```python
from build123d import *

# Parameters (mm, degrees)
ESQUISSE2_W              = 290
ESQUISSE2_H              = 184.53
BOSS_EXTRU_1_DEPTH       = 10
ESQUISSE9_R              = 2
ENL_V_MAT_EXTRU_7_DEPTH  = 10
ESQUISSE12_R             = 2
ENL_V_MAT_EXTRU_10_DEPTH = 10
ENL_V_MAT_EXTRU_12_DEPTH = 10
ENL_V_MAT_EXTRU_13_DEPTH = 10
CONG_1_R                 = 30
CONG_2_R                 = 30
ESQUISSE16_R             = 6
ENL_V_MAT_EXTRU_14_DEPTH = 5


with BuildPart() as part:
    # Esquisse2 → Boss.-Extru.1 (new body)
    with BuildSketch(Plane(origin=(0, 0, 0), x_dir=(1, 0, 0), z_dir=(0, 1, 0))):
        with Locations((145, 92.265)):
            Rectangle(ESQUISSE2_W, ESQUISSE2_H)
    extrude(amount=BOSS_EXTRU_1_DEPTH)

    # Esquisse9 → Enlèv. mat.-Extru.7 (cut)
    with BuildSketch(Plane(origin=(0, 10, 0), x_dir=(1, 0, 0), z_dir=(0, 1, 0))):
        with Locations((45, 50)):
            Circle(ESQUISSE9_R)
        with Locations((245, 50)):
            Circle(ESQUISSE9_R)
    extrude(amount=-ENL_V_MAT_EXTRU_7_DEPTH, mode=Mode.SUBTRACT)

    # Esquisse12 → Enlèv. mat.-Extru.10 (cut)
    with BuildSketch(Plane.XZ):
        with Locations((10, -165)):
            Circle(ESQUISSE12_R)
        with Locations((280, -165)):
            Circle(ESQUISSE12_R)
    extrude(amount=-ENL_V_MAT_EXTRU_10_DEPTH, mode=Mode.SUBTRACT)

    # Esquisse14 → Enlèv. mat.-Extru.12 (cut)
    with BuildSketch(Plane(origin=(0, 10, 0), x_dir=(1, 0, 0), z_dir=(0, 1, 0))):
        with BuildLine():
            Line((0, 184.53), (0, 165))
            ThreePointArc((0, 165), (2.928932188, 172.071067812), (10, 175))
            Line((10, 175), (280, 175))
            ThreePointArc((280, 175), (287.071067812, 172.071067812), (290, 165))
            Line((290, 165), (290, 184.53))
            Line((290, 184.53), (0, 184.53))
        make_face()
        with BuildLine():
            Line((245, 5), (45, 5))
            ThreePointArc((45, 5), (13.180194847, 18.180194847), (0, 50))
            Line((0, 50), (0, 0))
            Line((0, 0), (290, 0))
            Line((290, 0), (290, 50))
            ThreePointArc((290, 50), (276.819805153, 18.180194847), (245, 5))
        make_face()
    extrude(amount=-ENL_V_MAT_EXTRU_12_DEPTH, mode=Mode.SUBTRACT)

    # Esquisse15 → Enlèv. mat.-Extru.13 (cut)
    with BuildSketch(Plane(origin=(0, 10, 0), x_dir=(1, 0, 0), z_dir=(0, 1, 0))):
        Polygon((245, 5), (203.974576033, 50), (86.025423967, 50), (45, 5), align=None)
    extrude(amount=-ENL_V_MAT_EXTRU_13_DEPTH, mode=Mode.SUBTRACT)

    # Congé1
    cong_1_edges = [part.edges().sort_by_distance(p)[0] for p in [
        (86.025423967, 5, -50),
        (203.974576033, 5, -50),
    ]]
    fillet(cong_1_edges, radius=CONG_1_R)

    # Congé2
    cong_2_edges = [part.edges().sort_by_distance(p)[0] for p in [
        (45, 5, -5),
        (245, 5, -5),
    ]]
    fillet(cong_2_edges, radius=CONG_2_R)

    # Esquisse16 → Enlèv. mat.-Extru.14 (cut)
    with BuildSketch(Plane.XZ):
        with Locations((45, -50)):
            Circle(ESQUISSE16_R)
        with Locations((245, -50)):
            Circle(ESQUISSE16_R)
        with Locations((280, -165)):
            Circle(ESQUISSE16_R)
        with Locations((10, -165)):
            Circle(ESQUISSE16_R)
    extrude(amount=-ENL_V_MAT_EXTRU_14_DEPTH, mode=Mode.SUBTRACT)


solid = part.part
```
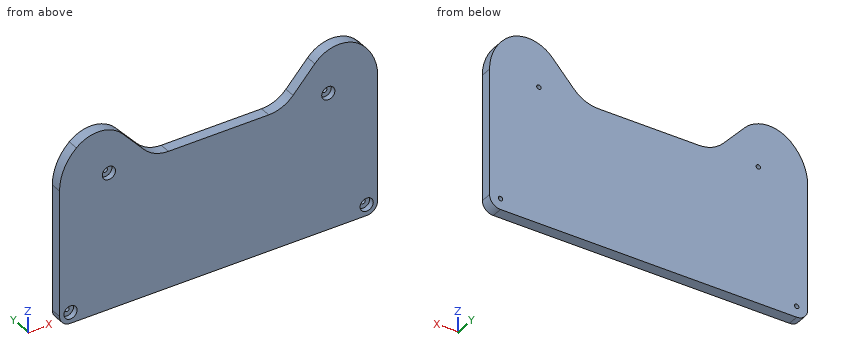
Here's how the part is built. I have some questions about the finished solid (model axes, mm). Coordinates: 2 decimals unless noted, no trailing zeros. Order: outer loops, then holes, each group sorted by start corner. A loop starts at its lowest first (then second) coordinate and runs counter-clockwise, first axis right, second up.
1) Imagine slicing it at B-B on x = 140.5. List the corners of the cut face in (y, z) for me.
2) Will these pins go through, and if not, where does the flat tip stop? pin 1 (11 mm diameter, centred on x = 45, z = -50, fed in from -Y); pin 2 (1.5 mm diameter, centred on x = 80, y = 5.5, fed in from +Z).
3) I need wall thicknesses on line 1 (Z direction, x = 122, y = 8.5); line 2 (X direction, y = 5.5, z = -19.5); line 3 (Z direction, x = 244, y = 8.5). Which ranges of each line are inside material? Lowest first, please.
4) Imagine slicing it at A-A on y = 7.25. List the corners of the cut face in (x, z) for me.
5) Imagine slicing it at C-C on x = 94. List the corners of the cut face in (y, z) for me, and give its area (3 significant figures).
Response values:
1. outline: (0, -175) - (10, -175) - (10, -50) - (0, -50) - close
2. pin 1: stops at y = 5
2. pin 2: stops at z = -42.34
3. line 1: z = -175 to -50
3. line 2: x = 11.91 to 58.22, 231.78 to 278.09
3. line 3: z = -175 to -51.73, -48.27 to -10.74
4. outline: (0, -165) arc R10 ccw to (10, -175) - (280, -175) arc R10 ccw to (290, -165) - (290, -50) arc R45 ccw to (274.61, -16.11) arc R30 ccw to (232.7, -18.49) - (212.9, -40.21) arc R30 cw to (190.73, -50) - (99.27, -50) arc R30 cw to (77.1, -40.21) - (57.3, -18.49) arc R30 ccw to (15.39, -16.11) arc R45 ccw to (0, -50) - close; hole circle Ø4 at (10, -165); hole circle Ø4 at (45, -50); hole circle Ø4 at (245, -50); hole circle Ø4 at (280, -165)
5. outline: (0, -175) - (10, -175) - (10, -49.53) - (0, -49.53) - close
5. area: 1,250 mm2
